Build history of the part. All positions in model axes, mm. Face numbers are marked on the shaded views. Round coordinates to 2 decimals unless told otherwise and drop trailing zeros. Write each loop counter-clockwise with the first axis right and the second up, starting at its lowest first coordinate (ties: lowest second). Pieces come first, ordered by that corner, then holes.
from build123d import *

# Parameters (mm, degrees)
F2_ANGLE_BACK  = 30
F2_ANGLE       = 60
F3_ANGLE_START = 150
F3_ANGLE       = 30


with BuildPart() as f1:
    # F0 (on Front) → F1 (revolve)
    with BuildSketch(Plane.XZ):
        Polygon((26.9527230412, 13.23380135), (26.9527230412, 39.6751612425), (23.2207458466, 39.6751612425), (23.2207458466, 15.7125871629), align=None)
        Polygon((26.9527230412, 7.6516205445), (26.9527230412, 13.23380135), (23.2207458466, 15.7125871629), (23.2207458466, 10.9555618837), align=None)
        Polygon((26.9527230412, -39.6751612425), (26.9527230412, 7.6516205445), (23.2207458466, 10.9555618837), (9.1962680429, 22.2483958323), (6.8564140238, 20.368527621), (23.2207458466, 0), (23.2207458466, -39.6751612425), align=None)
    revolve(axis=Axis((0, 0, 5.4553020746), (0, 0, -1)))

    # F0 (on Front) → F2 (revolve, cut)
    with BuildSketch(Plane.XZ, mode=Mode.PRIVATE) as f2_sk:
        Polygon((26.9527230412, 7.6516205445), (26.9527230412, 13.23380135), (23.2207458466, 15.7125871629), (23.2207458466, 10.9555618837), align=None)
    revolve(f2_sk.sketch.rotate(Axis((0, 0, 5.4553020746), (0, 0, 1)), -F2_ANGLE_BACK), axis=Axis((0, 0, 5.4553020746), (0, 0, 1)), revolution_arc=F2_ANGLE, mode=Mode.SUBTRACT)

    # F0 (on Front) → F3 (revolve, cut)
    with BuildSketch(Plane.XZ, mode=Mode.PRIVATE) as f3_sk:
        Polygon((26.9527230412, 7.6516205445), (26.9527230412, 13.23380135), (23.2207458466, 15.7125871629), (23.2207458466, 10.9555618837), align=None)
    revolve(f3_sk.sketch.rotate(Axis((0, 0, 5.4553020746), (0, 0, 1)), F3_ANGLE_START), axis=Axis((0, 0, 5.4553020746), (0, 0, 1)), revolution_arc=F3_ANGLE, mode=Mode.SUBTRACT)


solid = f1.part
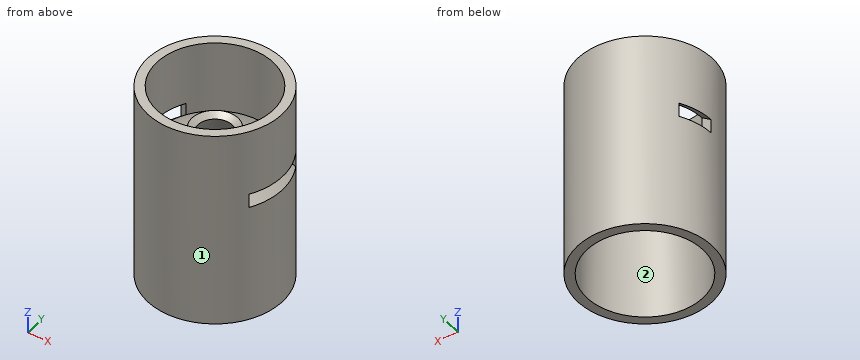
1) Pin check, flat tips, straight feed: pin 1 Ø3 at (x, y) = (12, -8) entering from +Z; pin 2 Ø12 at (x, z) = (11.5, -16) entering from +Y; pin 3 Ø3 at (x, z) = (-25.5, 12.5) entering from +Y; pin 4 Ø6 at (x, y) = (-8, 20.5) entering from +Z. Stop position of each tip, or through.
Results:
pin 1: stops at z = 19.25
pin 2: stops at y = 26.39
pin 3: stops at y = 11.88
pin 4: stops at z = 39.68
2) Wall check: L1, parallel to X at y = 0, z = -20; L2, parallel to X at y = -5.5, z = 20; L3, parallel to Y at x = 6.5, z = 17. Give the ranges that are in metal, low to high.
Results:
L1: x = -26.95 to -23.22, 23.22 to 26.95
L2: x = -26.39 to -22.56, -10.65 to -4.57, 4.57 to 10.65, 22.56 to 26.39
L3: y = -26.16 to -22.29, -14.31 to -7.01, 7.01 to 14.31, 22.29 to 26.16
3) Slice it at C-C (y = -1.5). Count the separate pieces of the cut face and the enclosed holes in it, plus the area to 3 significant figures.
Results:
separate pieces: 3
enclosed holes: 0
area: 807 mm2
4) Slice it at D-D (z = 28). Write the cut outline in (x, y), plus the area to 3 significant figures.
Results:
outline: circle Ø53.91 at (0, 0); hole circle Ø46.44 at (0, 0)
area: 588 mm2
5) Slice it at B-B (x = 0). Write the cut outline in (y, z).
Results:
outline: (-26.95, -39.68) - (-23.22, -39.68) - (-23.22, 0) - (-6.86, 20.37) - (-9.2, 22.25) - (-23.22, 10.96) - (-23.22, 39.68) - (-26.95, 39.68) - close; (6.86, 20.37) - (23.22, 0) - (23.22, -39.68) - (26.95, -39.68) - (26.95, 39.68) - (23.22, 39.68) - (23.22, 10.96) - (9.2, 22.25) - close
6) Slice it at A-A (z = 9.5). Write the cut outline in (x, y).
Results:
outline: (-26.95, 0) arc R26.95 ccw to (23.34, -13.48) - (21.53, -12.43) arc R24.86 ccw to (21.53, 12.43) - (23.34, 13.48) arc R26.95 ccw to (-23.34, 13.48) - (-21.53, 12.43) arc R24.86 ccw to (-24.86, 0) - close; hole circle Ø31.18 at (0, 0)
7) Mould opens along Y. For the marked faces 1 and 2 say: released by +Y, released by -Y, zero draft, split by the parting line, or undercut.
Results:
face 1: split by the parting line
face 2: undercut
